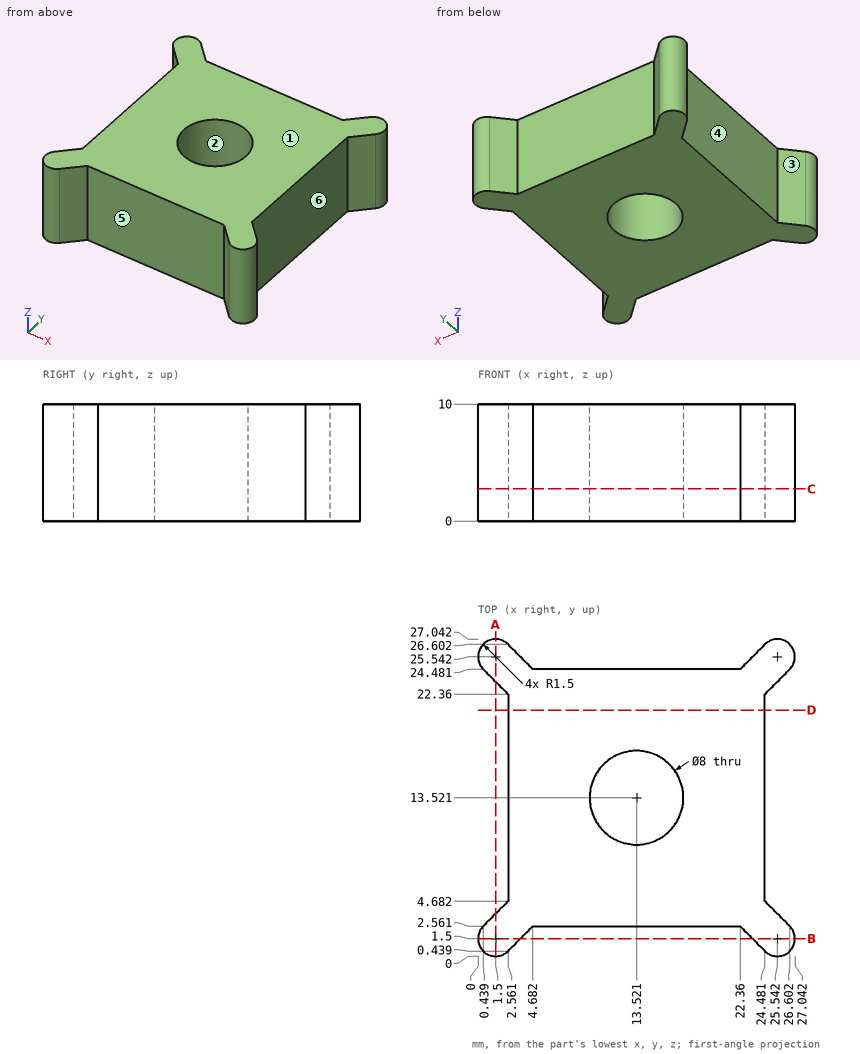
Geometry check sheet. Reference: drawing and pictorial views, mm from the part's lowest x, y, z. A direction names the side the tool comes from. Coordinates: 2 decimals unless noted, no trailing zeros. Order: outer loops, then holes, each group sorted by start corner. A loop starts at its lowest first (then second) coordinate and runs counter-clockwise, first axis right, second up. Notation, with made-up numbers: (15.25, -1) -> (71.25, -1) arc R19 ccw to (71.25, 26) -> close; hole circle Ø11 at (2.5, -9). An arc over 180 degrees is marked (long way). Put each result on its own line as item: value. Start each with the question number.
1) Cross-section at C-C (z = 2.75). Enter the section's corners in (x, y).
2) Material ranges on L1, parallel to Y at x = 5.5, z = 7; L2, parallel to X at y = 24.75, z = 7 (1 decimal); L3, parallel to Y at x = 14.75, z = 4 (1 decimal), recorded low to high.
3) Cross-section at A-A (x = 1.5). Enter the section's corners in (y, z).
4) Cross-section at D-D (y = 21). Enter the section's corners in (x, z).
5) Go/stop test with flat-tipped pins: pin 1 (3 mm diameter, centred on y = 10.5, z = 6.5, fed in from -X); pin 2 (2 mm diameter, centred on y = 17, z = 7.5, fed in from +X); pin 3 (1 mm diameter, centred on y = 23, z = 1.5, fed in from +X). Record where each tip stops, or that it passes through.
6) Release check for a two-part mould opening along X. For the marked faces 1, 2 and 3 record: pulls with the +X half, pulls with the -X half, needs draft (parallel to the pull), parting line crosses it, or undercut.
7) Tool access check on the marked faces 4, 5 and 6. Record the directions out of +Z, -Z, +X, -X, +Y, -Y that give a thin tool (end or side, any length) a straight path to the whole face; none if there is none.
Geometry check:
1. outline: (0.44, 2.56) arc R1.5 ccw to (2.56, 0.44) -> (4.68, 2.56) -> (22.36, 2.56) -> (24.48, 0.44) arc R1.5 ccw to (26.6, 2.56) -> (24.48, 4.68) -> (24.48, 22.36) -> (26.6, 24.48) arc R1.5 ccw to (24.48, 26.6) -> (22.36, 24.48) -> (4.68, 24.48) -> (2.56, 26.6) arc R1.5 ccw to (0.44, 24.48) -> (2.56, 22.36) -> (2.56, 4.68) -> close; hole circle Ø8 at (13.52, 13.52)
2. L1: y = 2.56 to 24.48
2. L2: x = 0.2 to 4.4, 22.6 to 26.8
2. L3: y = 2.6 to 9.7, 17.3 to 24.5
3. outline: (0, 0) -> (3.62, 0) -> (3.62, 10) -> (0, 10) -> close; (23.42, 0) -> (27.04, 0) -> (27.04, 10) -> (23.42, 10) -> close
4. outline: (2.56, 0) -> (24.48, 0) -> (24.48, 10) -> (2.56, 10) -> close
5. pin 1: stops at x = 2.56
5. pin 2: stops at x = 24.48
5. pin 3: stops at x = 25.62
6. face 1: needs draft
6. face 2: undercut
6. face 3: pulls with the -X half
7. face 4: +Z, -Z, -X
7. face 5: +Z, -Z, -Y
7. face 6: +Z, -Z, +X
